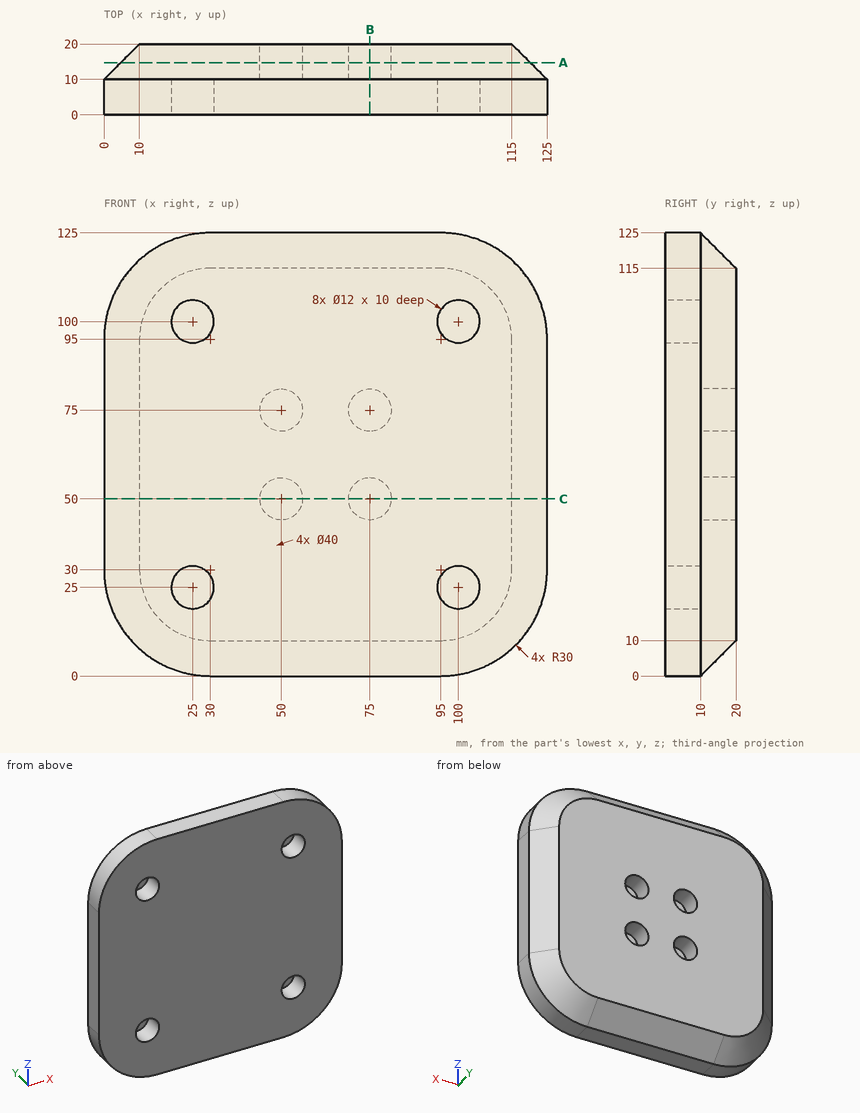
Here's the drawing with two shaded views (mm, measured from the low corner). I have some questions. Give positions to 0.01 mm unless a question says otherwise; leave off trailing zeros. Write each loop counter-clockwise with the first axis right and the second up, starting at its lowest first coordinate (ties: lowest second). Pieces come first, ordered by that corner, then holes. Notation, with made-up numbers: (82, 16) -> (114, 16) arc R14 cw to (114, 25) -> close; hole circle Ø10 at (56.5, 71.5). An arc over 180 degrees is marked (long way). Use one line per item in the form item = value.
1) Suppose I cut it at A-A (y = 14.75). Please give me the cut outline in (x, z).
Verdict:
outline = (4.75, 30) arc R25.25 ccw to (30, 4.75) -> (95, 4.75) arc R25.25 ccw to (120.25, 30) -> (120.25, 95) arc R25.25 ccw to (95, 120.25) -> (30, 120.25) arc R25.25 ccw to (4.75, 95) -> close; hole circle Ø12 at (50, 50); hole circle Ø12 at (50, 75); hole circle Ø12 at (75, 50); hole circle Ø12 at (75, 75)
2) Suppose I cut it at C-C (z = 50). Please give me the cut outline in (x, y), and give its area (3 significant figures).
Verdict:
outline = (0, 0) -> (125, 0) -> (125, 10) -> (115, 20) -> (81, 20) -> (81, 10) -> (69, 10) -> (69, 20) -> (56, 20) -> (56, 10) -> (44, 10) -> (44, 20) -> (10, 20) -> (0, 10) -> close
area = 2,160 mm2
3) Suppose I cut it at B-B (x = 75). Please give me the cut outline in (y, z).
Verdict:
outline = (0, 0) -> (10, 0) -> (20, 10) -> (20, 44) -> (10, 44) -> (10, 56) -> (20, 56) -> (20, 69) -> (10, 69) -> (10, 81) -> (20, 81) -> (20, 115) -> (10, 125) -> (0, 125) -> close
4) I'm going to push flat-ended pins straight in: pin 1 (2 mm diameter, centred on y = 15, z = 87.5, fed in from -X); pin 2 (6 mm diameter, centred on x = 102, z = 27, fed in from -Y); pin 3 (12 mm diameter, centred on x = 92, y = 16.5, fed in from +Z). Where does each tip first touch, or does it pass through?
Verdict:
pin_1 = 4
pin_2 = 10
pin_3 = 124.5
5) If I drill on L1, parallel to Z at x = 96.5, y = 4.5; L2, parallel to X at y = 6, z = 25; L3, parallel to X at y = 7.75, z = 103.5, over which ranges is the centre line in solid material (lowest first)? Write a range as [from, to].
Verdict:
L1 = [0.04, 20.13], [29.87, 95.13], [104.87, 124.96]
L2 = [0.42, 19], [31, 94], [106, 124.58]
L3 = [1.23, 20.13], [29.87, 95.13], [104.87, 123.77]
